from build123d import *

# Parameters (mm, degrees)
SKETCH_1_R          = 37.5
EXTRUDE_1_DEPTH     = 25.24
SKETCH_2_R          = 4
SKETCH_2_R_2        = 3
EXTRUDE_2_DEPTH     = 12
CUT_EXTRUDE_1_REACH = 60.733
SKETCH_3_R          = 3


with BuildPart() as part:
    # 草图1 → 凸台-拉伸1 (new body)
    with BuildSketch(Plane(origin=(0, 0, 0), x_dir=(1, 0, 0), z_dir=(0, 1, 0))):
        with Locations(Location((0, 0, 0), (0, 0, 270))):
            Circle(SKETCH_1_R)
    extrude(amount=EXTRUDE_1_DEPTH)

    # 草图2 → 凸台-拉伸2 (add)
    with BuildSketch(Plane(origin=(0, 25.24, 0), x_dir=(1, 0, 0), z_dir=(0, 1, 0))):
        with Locations(Location((0, 0, 0), (0, 0, 270))):
            Circle(SKETCH_2_R)
        with Locations(Location((0, 0, 0), (0, 0, 270))):
            Circle(SKETCH_2_R_2, mode=Mode.SUBTRACT)
    extrude(amount=EXTRUDE_2_DEPTH)

    # 草图3 → 切除-拉伸1 (cut, up to next)
    with BuildSketch(Plane(origin=(0, 25.24, 0), x_dir=(1, 0, 0), z_dir=(0, 1, 0)), mode=Mode.PRIVATE) as cut_extrude_1_sk1:
        with Locations(Location((0, 0, 0), (0, 0, 270))):
            Circle(SKETCH_3_R)
    cut_extrude_1_tool1 = extrude(cut_extrude_1_sk1.sketch, amount=-CUT_EXTRUDE_1_REACH, mode=Mode.PRIVATE) & part.part
    add(cut_extrude_1_tool1.solids().sort_by_distance((0, 25.24, 0))[0], mode=Mode.SUBTRACT)


solid = part.part
For this review, take the finished solid that the model builds, in its own axes (mm). A direction names the side the tool comes from. Coordinates: 2 decimals unless noted, no trailing zeros. Write each loop counter-clockwise with the first axis right and the second up, starting at its lowest first coordinate (ties: lowest second). Pieces come first, ordered by that corner, then holes. Notation, with made-up numbers: (35, -26) -> (63, -26) arc R26 ccw to (63, 10) -> close; hole circle Ø10 at (78.5, 66.25). An arc over 180 degrees is marked (long way). Write each question's results on one line, items separated by ' | '. Start each with the question number.
1) Consider section B-B (z = 0). Write out the cut boundary in (x, y), plus the area to 3 significant figures.
2) Insertion check: pin 1 (1.5 mm diameter, centred on x = -5, y = 22, fed in from -Z); pin 2 (12 mm diameter, centred on x = -3, z = -12, fed in from +Y); pin 3 (5 mm diameter, centred on x = 0, z = 0, fed in from +Y); pin 4 (3 mm diameter, centred on y = 14, z = 9, fed in from -X). Each pin has a flat end and moves straight along its axis. Give the tip position at first contact, or say it passes through.
3) Consider section A-A (x = 0). Write out the cut boundary in (y, z), plus the area to 3 significant figures.
4) For faces 1 (the face through (-3.905, 31.156, -0.867)), 2 (the face through (3, 37.24, 1)), list the 3-axis set-ups (+Z, -Z, +X, -X, +Y, -Y) from which the entire face can be reached by the end or side of a thin tool; tool diameter is ignored.
5) Wall thickness on L1, parallel to X at y = 31, z = 0; L2, parallel to X at y = 19, z = 0; L3, parallel to Y at x = 1, z = 30.5: over which ranges is each line inside the solid? List them lowest first. Write a range as [from, to].
6) Consider section D-D (z = 30). Write out the cut boundary in (x, y), plus the area to 3 significant figures.
7) Consider section C-C (y = 29.5). Write out the cut boundary in (x, z).
Geometry says:
1) outline: (-37.5, 0) -> (-3, 0) -> (-3, 37.24) -> (-4, 37.24) -> (-4, 25.24) -> (-37.5, 25.24) -> close; (3, 0) -> (37.5, 0) -> (37.5, 25.24) -> (4, 25.24) -> (4, 37.24) -> (3, 37.24) -> close | area: 1,770 mm^2
2) pin 1: z = -37.26 | pin 2: y = 25.24 | pin 3: through | pin 4: x = -36.74
3) outline: (0, -37.5) -> (25.24, -37.5) -> (25.24, -4) -> (37.24, -4) -> (37.24, -3) -> (0, -3) -> close; (0, 3) -> (37.24, 3) -> (37.24, 4) -> (25.24, 4) -> (25.24, 37.5) -> (0, 37.5) -> close | area: 1,770 mm^2
4) face 1: +Y | face 2: +Z, -Z, +X, -X, +Y
5) L1: [-4, -3], [3, 4] | L2: [-37.5, -3], [3, 37.5] | L3: [0, 25.24]
6) outline: (-22.5, 0) -> (22.5, 0) -> (22.5, 25.24) -> (-22.5, 25.24) -> close | area: 1,140 mm^2
7) outline: circle Ø8 at (0, 0); hole circle Ø6 at (0, 0)
